The listing builds one solid part. Answer for the finished solid, in the listing's coordinates (mm). Coordinates: 2 decimals unless noted, no trailing zeros. Write each loop counter-clockwise with the first axis right and the second up, starting at its lowest first coordinate (ties: lowest second). Pieces come first, ordered by that corner, then holes.
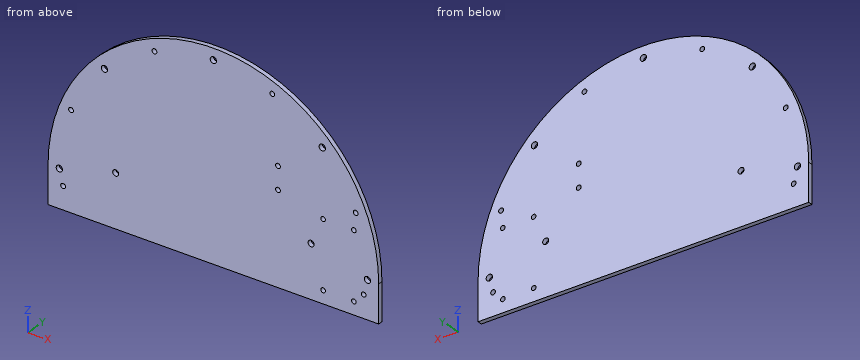
from build123d import *

# Parameters (mm, degrees)
EXTRUDE_1_DEPTH     = 3
SKETCH_2_W          = 220
SKETCH_2_H          = 200
CUT_EXTRUDE_1_DEPTH = 167.535281547
SKETCH_3_R          = 2
SKETCH_3_R_2        = 2.1
SKETCH_3_R_3        = 1.6
CUT_EXTRUDE_2_DEPTH = 10
SKETCH_4_R          = 1.6
CUT_EXTRUDE_3_DEPTH = 156.592416268
SKETCH_4_3_R        = 1.6
SKETCH_4_3_R_2      = 1.55
CUT_EXTRUDE_4_DEPTH = 10


with BuildPart() as part:
    # Sketch 1 → Extrude 1 (new body)
    with BuildSketch(Plane(origin=(0, 0, 0), x_dir=(1, 0, 0), z_dir=(0, 1, 0))):
        with BuildLine():
            Line((-110, 0), (-110, 125))
            Line((-110, 125), (110, 125))
            Line((110, 125), (110, 0))
            ThreePointArc((110, 0), (0, -110), (-110, 0))
        make_face()
    extrude(amount=EXTRUDE_1_DEPTH)

    # Sketch 2 → Cut-Extrude 1 (cut, through all)
    with BuildSketch(Plane(origin=(0, 3, 0), x_dir=(1, 0, 0), z_dir=(0, 1, 0))):
        with Locations((0, 125)):
            Rectangle(SKETCH_2_W, SKETCH_2_H)
    extrude(amount=-CUT_EXTRUDE_1_DEPTH, mode=Mode.SUBTRACT)

    # Sketch 3 → Cut-Extrude 2 (cut)
    with BuildSketch(Plane(origin=(0, 3, 0), x_dir=(1, 0, 0), z_dir=(0, 1, 0))):
        with Locations(Location((-65, -10, 0), (0, 0, 270))):
            Circle(SKETCH_3_R)
        with Locations(Location((65, -10, 0), (0, 0, 270))):
            Circle(SKETCH_3_R)
        with Locations(Location((0, -102.5, 0), (0, 0, 270))):
            Circle(SKETCH_3_R_2)
        with Locations(Location((-72.478445072, -72.478445072, 0), (0, 0, 270))):
            Circle(SKETCH_3_R_2)
        with Locations(Location((-102.5, 0, 0), (0, 0, 270))):
            Circle(SKETCH_3_R_2)
        with Locations(Location((102.5, 0, 0), (0, 0, 270))):
            Circle(SKETCH_3_R_2)
        with Locations(Location((72.478445072, -72.478445072, 0), (0, 0, 270))):
            Circle(SKETCH_3_R_2)
        with Locations(Location((-94.697652082, -39.225051817, 0), (0, 0, 270))):
            Circle(SKETCH_3_R_3)
        with Locations(Location((94.697652082, -39.225051817, 0), (0, 0, 270))):
            Circle(SKETCH_3_R_3)
        with Locations(Location((39.225051817, -94.697652082, 0), (0, 0, 270))):
            Circle(SKETCH_3_R_3)
        with Locations(Location((-39.225051817, -94.697652082, 0), (0, 0, 270))):
            Circle(SKETCH_3_R_3)
    extrude(amount=-CUT_EXTRUDE_2_DEPTH, mode=Mode.SUBTRACT)

    # Sketch 4 → Cut-Extrude 3 (cut, through all)
    with BuildSketch(Plane(origin=(0, 3, 0), x_dir=(1, 0, 0), z_dir=(0, 1, 0))):
        with Locations(Location((-100, 10, 0), (0, 0, 270))):
            Circle(SKETCH_4_R)
        with Locations(Location((100, 10, 0), (0, 0, 90))):
            Circle(SKETCH_4_R)
    extrude(amount=-CUT_EXTRUDE_3_DEPTH, mode=Mode.SUBTRACT)

    # Sketch 4_3 → Cut-Extrude 4 (cut)
    with BuildSketch(Plane(origin=(0, 3, 0), x_dir=(1, 0, 0), z_dir=(0, 1, 0))):
        with Locations(Location((-100, 10, 0), (0, 0, 270))):
            Circle(SKETCH_4_3_R)
        with Locations(Location((100, 10, 0), (0, 0, 90))):
            Circle(SKETCH_4_3_R)
        with Locations(Location((43, -36, 0), (0, 0, 270))):
            Circle(SKETCH_4_3_R)
        with Locations(Location((43, -51, 0), (0, 0, 270))):
            Circle(SKETCH_4_3_R)
        with Locations(Location((73, -28, 0), (0, 0, 270))):
            Circle(SKETCH_4_3_R_2)
        with Locations(Location((93.5, -28, 0), (0, 0, 270))):
            Circle(SKETCH_4_3_R_2)
        with Locations(Location((93.5, 16.5, 0), (0, 0, 270))):
            Circle(SKETCH_4_3_R_2)
        with Locations(Location((73, 16.5, 0), (0, 0, 270))):
            Circle(SKETCH_4_3_R_2)
    extrude(amount=-CUT_EXTRUDE_4_DEPTH, mode=Mode.SUBTRACT)


solid = part.part
Q1. The part is cut by section B-B, the plane y = 0.6. State how many separate pieces and enclosed holes the cut face has, then the cut area to 3 significant figures.
Answers below:
separate pieces: 1
enclosed holes: 19
area: 24,300 mm2
Q2. Find the intervals of material crossed by probe 1 along X at (y, z) = (0.9, -16.5); probe 2 along X at (y, z) = (1.75, 72.5); probe 3 along Z at (x, y) = (94.5, 1.9), in increasing order.
Answers below:
probe 1: x = -110 to 71.45, 74.55 to 91.95, 95.05 to 110
probe 2: x = -82.73 to -74.58, -70.38 to 70.38, 74.58 to 82.73
probe 3: z = -25 to -17.68, -15.32 to 26.82, 29.18 to 37.64, 40.81 to 56.3
Q3. Given pin 1 (1 mm diameter, centred on y = 2.5, z = 74.5, fed in from +X), flat-ended and moving along its own axis, determine where the tip first touches the part or whether it passes through.
Answers below:
pin 1: stops at x = 81.39
Q4. The part is cut by section A-A, the plane x = 0. Write down the section's boundary in (y, z).
Answers below:
outline: (0, -25) - (3, -25) - (3, 100.4) - (0, 100.4) - close; (0, 104.6) - (3, 104.6) - (3, 110) - (0, 110) - close
Q5. The part is cut by section C-C, the plane z = 91. Write down the section's boundary in (x, y), then the cut area to 3 significant figures.
Answers below:
outline: (-61.8, 0) - (61.8, 0) - (61.8, 3) - (-61.8, 3) - close
area: 371 mm2
Q6. The part is cut by section D-D, the plane x = 85. Write down the section's boundary in (y, z).
Answers below:
outline: (0, -25) - (3, -25) - (3, 69.82) - (0, 69.82) - close
